Verification items for the finished model (mm, model axes). Face numbers are marked on the shaded views. A direction names the side the tool comes from. Round coordinates to 2 decimals unless told otherwise and drop trailing zeros. Order: outer loops, then holes, each group sorted by start corner. A loop starts at its lowest first (then second) coordinate and runs counter-clockwise, first axis right, second up. Notation, with made-up numbers: (-23.75, -5) -> (27.25, -5) arc R12 ccw to (27.25, 6) -> close; hole circle Ø1 at (19.25, 75.25). An arc over 180 degrees is marked (long way). Put each result on its own line as item: value.
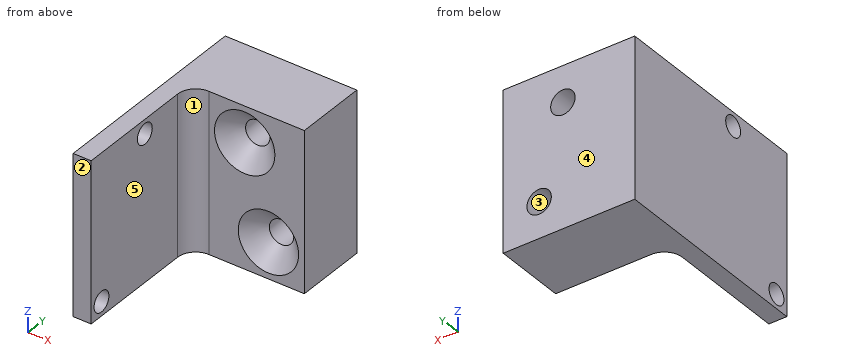
Autodesk Inventor part; units mm, degrees
ref_plane "YZ Plane" through (0, 0, 0) normal (1, 0, 0) x (0, 1, 0)
ref_plane "XZ Plane" through (0, 0, 0) normal (0, 1, 0) x (-1, 0, 0)
ref_plane "XY Plane" through (0, 0, 0) normal (0, 0, 1) x (1, 0, 0)
sketch "Sketch1" plane through (0, 0, 0) normal (0, 0, 1) x (1, 0, 0)
  line L0 (0, 0) -> (3.175, 0)
  line L1 (3.175, 0) -> (3.175, 24.13)
  line L2 (0, 36.83) -> (0, 0)
  line L3 (23.2455, 36.83) -> (23.2455, 24.13)
  line L4 (23.2455, 24.13) -> (3.175, 24.13)
  line L5 (0, 36.83) -> (23.2455, 36.83)
  dimension "d0" = 12.7
  dimension "d1" = 3.175
  dimension "d2" = 36.83
extrude "Extrusion1" add sketch "Sketch1" along normal blind 28.194
sketch "Sketch2" plane through (3.175, 0, 0) normal (1, 0, 0) x (0, 0, -1)
  circle A0 centre (-2.5, 2.5) radius 1.8
  circle A1 centre (-25.694, 13) radius 1.8
  line L0 (0, 0) -> (0, 24.13)
  line L1 (0, 0) -> (-28.194, 0)
  line L2 (-28.194, 0) -> (-28.194, 24.13)
  dimension "d5" = 3.6
  dimension "d6" = 3.6
  dimension "d7" = 2.5
  dimension "d8" = 2.5
  dimension "d9" = 2.5
  dimension "d10" = 13
extrude "Extrusion2" cut sketch "Sketch2" against normal blind 28.194
fillet "Fillet1" radius 3.175 1 edges at (3.175, 24.13, 14.097)
sketch "Sketch3" plane through (23.2455, 24.13, 0) normal (0, -1, 0) x (1, 0, 0)
  line L0 (-16.8955, 0) -> (-16.8955, 28.194)
  line L1 (-16.8955, 0) -> (0, 0)
  line L2 (0, 0) -> (0, 28.194)
  line L3 (-16.8955, 28.194) -> (0, 28.194)
  circle A0 centre (-10.5455, 21.844) radius 2.159
  circle A1 centre (-6.35, 6.35) radius 2.159
  point P0 (-23.2455, 0)
  dimension "d14" = 4.318
  dimension "d15" = 4.318
  dimension "d16" = 6.35
  dimension "d18" = 6.35
  dimension "d19" = 6.35
  dimension "d20" = 6.35
extrude "Extrusion3" cut sketch "Sketch3" against normal blind 28.194 contours A0 | A1
chamfer "Chamfer1" distance 3.175 angle 45 2 edges at (14.7365, 24.13, 6.35) (10.541, 24.13, 21.844)
properties part number "Limit Switch Top V1_3DPrint"
Item 1: Sectioned sample at B-B, the plane y = 2.5. Record the boundary of the cut face in (x, z) (3 decimals), then the cut area to 3 significant figures.
Geometry check:
outline: (0, 0) -> (3.175, 0) -> (3.175, 0.7) -> (0, 0.7) -> close; (0, 4.3) -> (3.175, 4.3) -> (3.175, 28.194) -> (0, 28.194) -> close
area: 78.1 mm2
Item 2: Material ranges on line 1 along Z through (x, y) = (12.7, 30) (3 decimals); line 2 along Y through (x, z) = (7, 13); line 3 along X through (y, z) = (5, 23.75) (3 decimals), recorded low to high.
Geometry check:
line 1: 0 to 19.685, 24.003 to 28.194
line 2: 24.13 to 36.83
line 3: 0 to 3.175
Item 3: Tool access check on the marked faces 4 and 5. Record the directions out of +Z, -Z, +X, -X, +Y, -Y that give a thin tool (end or side, any length) a straight path to the whole face; none if there is none.
Geometry check:
face 4: +Z, -Z, +X, -X, +Y
face 5: +Z, -Z, +X, -Y
Item 4: Release check for a two-part mould opening along X. For the marked faces 1, 2 and 3 record: pulls with the +X half, pulls with the -X half, needs draft (parallel to the pull), parting line crosses it, or undercut.
Geometry check:
face 1: pulls with the +X half
face 2: needs draft
face 3: undercut
Item 5: Depth check by flat-ended pin: pin 1 Ø6 at (y, z) = (2.5, 2.5) entering from +X (3 decimals); pin 2 Ø5 at (x, z) = (17, 19.5) entering from -Y; pin 3 Ø7 at (x, z) = (16.9, 6.35) entering from -Y. Enter the tip coordinate at first touch or a pass-through.
Geometry check:
pin 1: x = 3.175
pin 2: y = 24.13
pin 3: y = 25.96
Item 6: Sectioned sample at C-C, the plane y = 20. Record the boundary of the cut face in (x, z) (3 decimals).
Geometry check:
outline: (0, 0) -> (3.175, 0) -> (3.175, 28.194) -> (0, 28.194) -> close
